from build123d import *

# Parameters (mm, degrees)
F0_W     = 140
F0_H     = 50
F0_R     = 1.75
F0_R_2   = 3.25
F0_R_3   = 2.5
F1_DEPTH = 8
F2_SIZE  = 3
F4_D     = 8.8


with BuildPart() as f1:
    # F0 (on Top) → F1 (new body)
    with BuildSketch(Plane.XY):
        Rectangle(F0_W, F0_H)
        with Locations((-62.4999959502, -16.0005345571)):
            Circle(F0_R, mode=Mode.SUBTRACT)
        with Locations((62.5, -15.968715623)):
            Circle(F0_R, mode=Mode.SUBTRACT)
        with Locations((-42, 15)):
            Circle(F0_R_2, mode=Mode.SUBTRACT)
        with Locations((-62.4999959502, 18.9994654429)):
            Circle(F0_R, mode=Mode.SUBTRACT)
        Circle(F0_R_3, mode=Mode.SUBTRACT)
        with Locations((42, 15)):
            Circle(F0_R_2, mode=Mode.SUBTRACT)
        with Locations((62.5, 19.031284377)):
            Circle(F0_R, mode=Mode.SUBTRACT)
    extrude(amount=F1_DEPTH)

    # F2
    f2_edges = [f1.edges().sort_by_distance(p)[0] for p in [
        (-70, -25, 4),
        (70, -25, 4),
        (70, 25, 4),
        (-70, 25, 4),
    ]]
    chamfer(f2_edges, length=F2_SIZE)

    # F4 (through all)
    with Locations(Plane.XY.offset(8)):
        with Locations((0, 0)):
            Hole(F4_D / 2)


solid = f1.part
Design review of the part built by this model. Coordinates are the model's own, in mm. Give positions to 0.01 mm unless a question says otherwise; leave off trailing zeros. Write each loop counter-clockwise with the first axis right and the second up, starting at its lowest first coordinate (ties: lowest second). Pieces come first, ordered by that corner, then holes. Notation, with made-up numbers: M 61.25,31.5 L 70.25,31.5 A24 ccw 70.25,61.5 Z; hole C -22,74.5 d2. An arc over 180 degrees is marked long. Answer as a JSON object with one key per item and string values. Group by question number.
1) We need section B-B (x = 62.5). Give the boundary of the cut face in (y, z).
2) We need section D-D (y = 0). Give the boundary of the cut face in (x, z).
3) We need section C-C (x = -42). Give the boundary of the cut face in (y, z).
4) Mouldability with a two-part tool opening along X and no side actions: class faces 1 (the face through (69, 23, 4)), 2 (the face through (-1, 25, 4)), 3 (the face through (-38.9, 15.98, 3.94)) as released by +X, released by -X, zero draft, split by the parting line, or undercut.
5) For line 1 along Y through (x, z) = (62.5, 2.5); line 2 along X through (y, z) = (19.5, 1.25); line 3 along X through (y, z) = (-14.5, 1.25), list the stretches that pass through material, from the lowest coordinate up.
6) We need section A-A (y = 15). Give the boundary of the cut face in (x, z), and give its area (3 significant figures).
Answer key:
{
 "1": {"outline": "M -25,0 L -17.72,0 L -17.72,8 L -25,8 Z; M -14.22,0 L 17.28,0 L 17.28,8 L -14.22,8 Z; M 20.78,0 L 25,0 L 25,8 L 20.78,8 Z"},
 "2": {"outline": "M -70,0 L -4.4,0 L -4.4,8 L -70,8 Z; M 4.4,0 L 70,0 L 70,8 L 4.4,8 Z"},
 "3": {"outline": "M -25,0 L 11.75,0 L 11.75,8 L -25,8 Z; M 18.25,0 L 25,0 L 25,8 L 18.25,8 Z"},
 "4": {"face 1": "released by +X", "face 2": "zero draft", "face 3": "undercut"},
 "5": {"line 1": "y = -25 to -17.72, -14.22 to 17.28, 20.78 to 25", "line 2": "x = -70 to -64.18, -60.82 to 60.81, 64.19 to 70", "line 3": "x = -70 to -63.4, -61.6 to 61.55, 63.45 to 70"},
 "6": {"outline": "M -70,0 L -45.25,0 L -45.25,8 L -70,8 Z; M -38.75,0 L 38.75,0 L 38.75,8 L -38.75,8 Z; M 45.25,0 L 70,0 L 70,8 L 45.25,8 Z", "area": "1,020 mm²"}
}
